Input: part model. Units: mm. Frame: model coordinates. Face numbers are marked on the shaded views. A direction names the side the tool comes from. Give positions to 0.01 mm unless a question says otherwise; leave off trailing zeros. Loops run counter-clockwise (first coordinate to the right, second up) from the corner with the lowest first, then second, coordinate; pieces in that order, holes last.
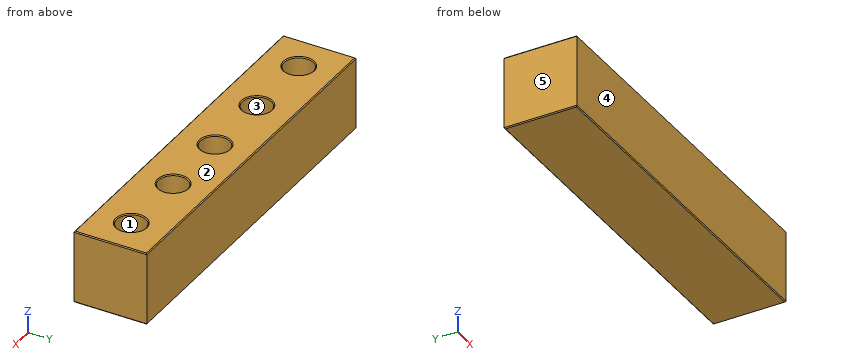
from build123d import *

# Parameters (mm, degrees)
EXPORT001_W     = 150
EXPORT001_H     = 30
EXPORT001_R     = 6
PAD_DEPTH       = 10
EXPORT002_W     = 150
EXPORT002_H     = 30
PAD001_DEPTH    = 20
CHAMFER_SIZE    = 0.4
CHAMFER001_SIZE = 0.4


with BuildPart() as part:
    # Export001 → Pad (new body)
    with BuildSketch(Plane.XY):
        with Locations((75, 0)):
            Rectangle(EXPORT001_W, EXPORT001_H)
        with Locations((15, 0)):
            Circle(EXPORT001_R, mode=Mode.SUBTRACT)
        with Locations((45, 0)):
            Circle(EXPORT001_R, mode=Mode.SUBTRACT)
        with Locations((75, 0)):
            Circle(EXPORT001_R, mode=Mode.SUBTRACT)
        with Locations((105, 0)):
            Circle(EXPORT001_R, mode=Mode.SUBTRACT)
        with Locations((135, 0)):
            Circle(EXPORT001_R, mode=Mode.SUBTRACT)
    extrude(amount=PAD_DEPTH)

    # Export002 → Pad001 (join)
    with BuildSketch(Plane.XY):
        with Locations((75, 0)):
            Rectangle(EXPORT002_W, EXPORT002_H)
    extrude(amount=-PAD001_DEPTH)

    # Chamfer
    chamfer_edges = [part.edges().sort_by_distance(p)[0] for p in [
        (75, 15, -20),
        (150, 0, -20),
        (75, -15, -20),
        (0, 0, -20),
    ]]
    chamfer(chamfer_edges, length=CHAMFER_SIZE)

    # Chamfer001
    chamfer001_edges = [part.edges().sort_by_distance(p)[0] for p in [
        (75, 15, 10),
        (150, 0, 10),
        (75, -15, 10),
        (0, 0, 10),
        (129, 0, 10),
        (99, 0, 10),
        (69, 0, 10),
        (39, 0, 10),
        (9, 0, 10),
    ]]
    chamfer(chamfer001_edges, length=CHAMFER001_SIZE)


solid = part.part
(1) Mould query, pull axis Y, two halves, no side actions, for the marked faces 3, 4 and 5. Classes: +Y half, -Y half, draft (parallel to the pull), parting line (faces both ways), or undercut.
Values follow:
face 3: undercut
face 4: -Y half
face 5: draft
(2) Cut plane A-A (z = 3). Return the cut outline in (x, y).
Values follow:
outline: (0, -15) - (150, -15) - (150, 15) - (0, 15) - close; hole circle Ø12 at (15, 0); hole circle Ø12 at (45, 0); hole circle Ø12 at (75, 0); hole circle Ø12 at (105, 0); hole circle Ø12 at (135, 0)
(3) Cut plane B-B (x = 45). Return the cut outline in (y, z), and give its area (3 significant figures).
Values follow:
outline: (-15, -19.6) - (-14.6, -20) - (14.6, -20) - (15, -19.6) - (15, 9.6) - (14.6, 10) - (6.4, 10) - (6, 9.6) - (6, 0) - (-6, 0) - (-6, 9.6) - (-6.4, 10) - (-14.6, 10) - (-15, 9.6) - close
area: 780 mm2
(4) Ray query, probe 1 along Y at (x, z) = (15, 7.5); probe 2 along X at (y, z) = (-4.5, 6); probe 3 along Z at (x, y) = (101, 0.5). Return the intervals inside material, ascending.
Values follow:
probe 1: y = -15 to -6, 6 to 15
probe 2: x = 0 to 11.03, 18.97 to 41.03, 48.97 to 71.03, 78.97 to 101.03, 108.97 to 131.03, 138.97 to 150
probe 3: z = -20 to 0
(5) Reachability of the marked faces 1 and 2 from +Z, -Z, +X, -X, +Y, -Y: full face, straight path, thin tool, end or side. Return the list, or none.
Values follow:
face 1: +Z
face 2: +Z, +X, -X, +Y, -Y
(6) Pin query (flat end, axial travel): pin 1 Ø9.5 at (x, y) = (14.5, 0) entering from +Z; pin 2 Ø1 at (x, y) = (41, -4) entering from +Z. Return the tip coordinate at first contact, or that it passes through.
Values follow:
pin 1: stops at z = 0
pin 2: stops at z = 9.76
